Could you check a few things on this model? Use its own coordinates, in mm. Face numbers are marked on the shaded views. A direction names the side the tool comes from. Round coordinates to 2 decimals unless told otherwise and drop trailing zeros. Loops run counter-clockwise (first coordinate to the right, second up) from the corner with the lowest first, then second, coordinate; pieces in that order, holes last.
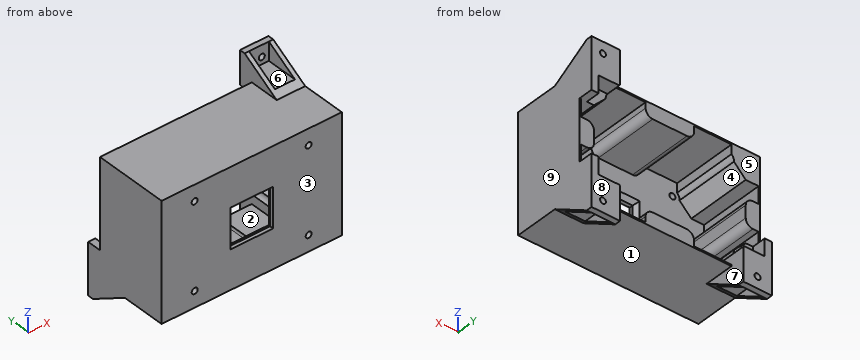
from build123d import *

# Parameters (mm, degrees)
SKETCH_1_W               = 126.5
SKETCH_1_H               = 82.5
SKETCH_1_R               = 2.1
SKETCH_1_W_2             = 30
SKETCH_1_H_2             = 28
EXTRUDE_2_DEPTH          = 6
CHAMFER_1_SIZE           = 2
CHAMFER_1_SIZE2          = 3.464101615
SKETCH_2_W               = 34
SKETCH_2_H               = 10
SKETCH_2_W_2             = 10
SKETCH_2_H_2             = 18.59934511
SKETCH_2_W_3             = 1
SKETCH_2_H_3             = 11.900654894
SKETCH_2_H_4             = 18.599345106
SKETCH_2_H_5             = 12
SKETCH_2_W_4             = 26.25
SKETCH_2_H_6             = 1
SKETCH_2_H_7             = 11.999999996
EXTRUDE_3_DEPTH          = 46
EXTRUDE_4_DEPTH          = 10
EXTRUDE_7_DEPTH          = 20
EXTRUDE_8_DEPTH          = 20
CUT_EXTRUDE_1_DEPTH      = 205.414906938
CUT_EXTRUDE_1_DEPTH_BACK = 205.414906938
SKETCH_6_R               = 2.1
SKETCH_7_W               = 14
SKETCH_7_H               = 13.763943164
SKETCH_7_H_2             = 13.67346934
SKETCH_7_H_3             = 14.015580363
SKETCH_7_H_4             = 13.891937121
CUT_EXTRUDE_2_DEPTH      = 58
FILLET_1_R               = 5
SKETCH_9_R               = 5
CUT_EXTRUDE_4_DEPTH      = 203.675736531


with BuildPart() as part:
    # Эскиз1 → Бобышка-Вытянуть2 (new body)
    with BuildSketch(Plane(origin=(0, 77.195974268, 0), x_dir=(1, 0, 0), z_dir=(0, 1, 0))):
        with Locations((64.808980694, -89.523129836)):
            Rectangle(SKETCH_1_W, SKETCH_1_H)
        with Locations(Location((24.808980694, -59.523129836, 0), (0, 0, 180))):
            Circle(SKETCH_1_R, mode=Mode.SUBTRACT)
        with Locations(Location((104.808980694, -59.523129836, 0), (0, 0, 180))):
            Circle(SKETCH_1_R, mode=Mode.SUBTRACT)
        with Locations(Location((104.808980694, -119.523129836, 0), (0, 0, 180))):
            Circle(SKETCH_1_R, mode=Mode.SUBTRACT)
        with Locations(Location((24.808980694, -119.523129836, 0), (0, 0, 180))):
            Circle(SKETCH_1_R, mode=Mode.SUBTRACT)
        with Locations((64.808980694, -89.523129836)):
            Rectangle(SKETCH_1_W_2, SKETCH_1_H_2, mode=Mode.SUBTRACT)
    extrude(amount=EXTRUDE_2_DEPTH)

    # Фаска1
    chamfer_1_edges = [part.edges().sort_by_distance(p)[0] for p in [
        (49.808980694, 83.195974268, 89.523129836),
        (64.808980694, 83.195974268, 103.523129836),
        (79.808980694, 83.195974268, 89.523129836),
        (64.808980694, 83.195974268, 75.523129836),
    ]]
    chamfer_1_side = [part.faces().sort_by_distance(p)[0] for p in [
        (64.808980694, 83.195974268, 49.78337816),
    ]]
    chamfer(chamfer_1_edges, length=CHAMFER_1_SIZE, length2=CHAMFER_1_SIZE2, reference=chamfer_1_side[0])

    # Эскиз2 → Бобышка-Вытянуть3 (add)
    with BuildSketch(Plane(origin=(0, 83.195974268, 0), x_dir=(1, 0, 0), z_dir=(0, 1, 0))):
        Polygon((1.558980694, -68.273129836), (11.558980694, -68.273129836), (21.558980694, -58.273129836), (21.558980694, -48.273129836), (1.558980694, -48.273129836), align=None)
        with Locations((64.808980694, -53.273129836)):
            Rectangle(SKETCH_2_W, SKETCH_2_H)
        Polygon((118.058980694, -68.273129836), (108.058980694, -58.273129836), (108.058980694, -48.273129836), (128.058980694, -48.273129836), (128.058980694, -68.273129836), align=None)
        with Locations((123.058980694, -89.473457285)):
            Rectangle(SKETCH_2_W_2, SKETCH_2_H_2)
        Polygon((108.058980694, -120.773129836), (118.058980694, -110.773129836), (128.058980694, -110.773129836), (128.058980694, -130.773129836), (108.058980694, -130.773129836), align=None)
        with Locations((64.808980694, -125.773129836)):
            Rectangle(SKETCH_2_W, SKETCH_2_H)
        Polygon((21.558980694, -130.773129836), (21.558980694, -120.773129836), (11.558980694, -110.773129836), (1.558980694, -110.773129836), (1.558980694, -130.773129836), align=None)
        with Locations((2.058980694, -74.223457283)):
            Rectangle(SKETCH_2_W_3, SKETCH_2_H_3)
        with Locations((6.558980694, -89.473457283)):
            Rectangle(SKETCH_2_W_2, SKETCH_2_H_4)
        with Locations((2.058980694, -104.773129836)):
            Rectangle(SKETCH_2_W_3, SKETCH_2_H_5)
        with Locations((34.683980694, -130.273129836)):
            Rectangle(SKETCH_2_W_4, SKETCH_2_H_6)
        with Locations((94.933980694, -130.273129836)):
            Rectangle(SKETCH_2_W_4, SKETCH_2_H_6)
        with Locations((127.558980694, -104.773129838)):
            Rectangle(SKETCH_2_W_3, SKETCH_2_H_7)
        with Locations((127.558980694, -74.223457283)):
            Rectangle(SKETCH_2_W_3, SKETCH_2_H_3)
        with Locations((94.933980694, -48.773129836)):
            Rectangle(SKETCH_2_W_4, SKETCH_2_H_6)
        with Locations((34.683980694, -48.773129836)):
            Rectangle(SKETCH_2_W_4, SKETCH_2_H_6)
    extrude(amount=EXTRUDE_3_DEPTH)

    # Эскиз3 → Бобышка-Вытянуть4 (add)
    with BuildSketch(Plane(origin=(0, 129.195974268, 0), x_dir=(1, 0, 0), z_dir=(0, 1, 0))):
        Polygon((6.558980694, -68.273129836), (6.558980694, -56.273129836), (21.558980694, -56.273129836), (21.558980694, -48.273129836), (1.558980694, -48.273129836), (1.558980694, -68.273129836), align=None)
        Polygon((123.058980694, -68.273129836), (123.058980694, -56.273129836), (108.058980694, -56.273129836), (108.058980694, -48.273129836), (128.058980694, -48.273129836), (128.058980694, -68.273129836), align=None)
        Polygon((123.058980694, -110.773129836), (123.058980694, -122.773129836), (108.058980694, -122.773129836), (108.058980694, -130.773129836), (128.058980694, -130.773129836), (128.058980694, -110.773129836), align=None)
    extrude(amount=EXTRUDE_4_DEPTH)

    # Эскиз4 → Бобышка-Вытянуть7 (add)
    with BuildSketch(Plane.ZY.offset(-1.558980694)):
        Polygon((48.273129836, 139.195974268), (48.273129836, 108.195974268), (32.273129836, 135.145974268), (32.273129836, 139.195974268), align=None)
    extrude(amount=-EXTRUDE_7_DEPTH)

    # Эскиз5 → Бобышка-Вытянуть8 (add)
    with BuildSketch(Plane(origin=(128.058980694, 0, 0), x_dir=(0, 0, -1), z_dir=(1, 0, 0))):
        Polygon((-130.773129836, 139.195974268), (-130.773129836, 108.145974268), (-146.773129836, 135.145974268), (-146.773129836, 139.195974268), align=None)
        Polygon((-48.273129836, 139.195974268), (-48.273129836, 108.195974268), (-32.273129836, 135.145974268), (-32.273129836, 139.195974268), align=None)
    extrude(amount=-EXTRUDE_8_DEPTH)

    # Эскиз6 → Вырез-Вытянуть1 (cut, two sides: drawn at the far end of the back side and taken through both)
    with BuildSketch(Plane(origin=(0, 139.195974268, 0), x_dir=(1, 0, 0), z_dir=(0, 1, 0)).offset(-CUT_EXTRUDE_1_DEPTH_BACK)):
        with Locations(Location((120.058980694, -40.273129836, 0), (0, 0, 90))):
            Circle(SKETCH_6_R)
        with Locations(Location((11.55898069, -40.273129836, 0), (0, 0, 180))):
            Circle(SKETCH_6_R)
        with Locations((11.55898069, -138.773129836)):
            Circle(SKETCH_6_R)
        with Locations(Location((120.058980694, -138.773129836, 0), (0, 0, 180))):
            Circle(SKETCH_6_R)
    extrude(amount=CUT_EXTRUDE_1_DEPTH + CUT_EXTRUDE_1_DEPTH_BACK, mode=Mode.SUBTRACT)

    # Эскиз7 → Вырез-Вытянуть2 (cut)
    with BuildSketch(Plane(origin=(0, 77.195974268, 0), x_dir=(-1, 0, 0), z_dir=(0, -1, 0))):
        with Locations((-11.558980694, -38.391158254)):
            Rectangle(SKETCH_7_W, SKETCH_7_H)
        with Locations((-118.058980694, -38.436395166)):
            Rectangle(SKETCH_7_W, SKETCH_7_H_2)
        with Locations((-118.058980694, -140.780920018)):
            Rectangle(SKETCH_7_W, SKETCH_7_H_3)
        with Locations((-11.558980694, -140.719098397)):
            Rectangle(SKETCH_7_W, SKETCH_7_H_4)
    extrude(amount=-CUT_EXTRUDE_2_DEPTH, mode=Mode.SUBTRACT)

    # Скругление1
    fillet_1_edges = [part.edges().sort_by_distance(p)[0] for p in [
        (81.808980694, 106.195974268, 120.773129836),
        (47.808980694, 106.195974268, 120.773129836),
        (11.558980694, 106.195974268, 98.773129836),
        (11.558980694, 106.195974268, 80.17378473),
        (47.808980694, 106.195974268, 58.273129836),
        (81.808980694, 106.195974268, 58.273129836),
        (118.058980694, 106.195974268, 80.17378473),
        (118.058980694, 106.195974268, 98.77312984),
    ]]
    fillet(fillet_1_edges, radius=FILLET_1_R)

    # Эскиз9 → Вырез-Вытянуть4 (cut, through all)
    with BuildSketch(Plane(origin=(0, 83.195974268, 0), x_dir=(1, 0, 0), z_dir=(0, 1, 0))):
        with Locations((24.808980694, -59.523129836)):
            Circle(SKETCH_9_R)
        with Locations((104.808980694, -59.523129836)):
            Circle(SKETCH_9_R)
        with Locations((104.808980694, -119.523129836)):
            Circle(SKETCH_9_R)
        with Locations((24.808980694, -119.523129836)):
            Circle(SKETCH_9_R)
    extrude(amount=CUT_EXTRUDE_4_DEPTH, mode=Mode.SUBTRACT)


solid = part.part
Item 1: If I drill on line 1 along X through (y, z) = (121, 73); line 2 along Z through (x, y) = (25.5, 109); line 3 along X through (y, z) = (126.5, 53), over which ranges is the centre line in solid material (lowest first)?
Results list:
line 1: x = 1.56 to 2.56, 127.06 to 128.06
line 2: z = 48.27 to 49.27, 129.77 to 130.77
line 3: x = 1.56 to 21.56, 47.81 to 81.81, 108.06 to 128.06
Item 2: For the marked faces 5, 6, 7, 8 and 9, which set-ups out of +Z, -Z, +X, -X, +Y, -Y let a thin tool reach every point of the face, with its end or its side?
Results list:
face 5: +Z, -X, +Y
face 6: +Z, -Y
face 7: +Y
face 8: +Z, -Z, +X, -X, +Y
face 9: +Z, -Z, +X, +Y, -Y
Item 3: If we section it at A-A, the plane z = 102: Please give me the cut outline in (x, y), then the cut area to 3 significant figures.
Results list:
outline: (1.56, 77.2) - (49.81, 77.2) - (49.81, 79.73) - (47.81, 83.2) - (2.56, 83.2) - (2.56, 129.2) - (1.56, 129.2) - close; (79.81, 77.2) - (128.06, 77.2) - (128.06, 129.2) - (127.06, 129.2) - (127.06, 83.2) - (81.81, 83.2) - (79.81, 79.73) - close
area: 664 mm2
Item 4: We'd pull the mould along Z, two halves only. Please class the marked faces 1, 2, 3 and 4: released by +Z, released by -Z, zero draft, split by the parting line, or undercut.
Results list:
face 1: released by -Z
face 2: undercut
face 3: zero draft
face 4: undercut
Item 5: If we section it at B-B, the plane x = 56.5: Please give me the cut outline in (y, z).
Results list:
outline: (77.2, 48.27) - (129.2, 48.27) - (129.2, 58.27) - (83.2, 58.27) - (83.2, 73.52) - (79.73, 75.52) - (77.2, 75.52) - close; (77.2, 103.52) - (79.73, 103.52) - (83.2, 105.52) - (83.2, 120.77) - (129.2, 120.77) - (129.2, 130.77) - (77.2, 130.77) - close
Item 6: Will these pins go through, and if not, where does the flat tip stop? pin 1 (6 mm diameter, centred on x = 96.5, y = 108, fed in from +Z); pin 2 (9.5 mm diameter, centred on x = 118.5, z = 114.5, fed in from +Y); pin 3 (11 mm diameter, centred on x = 125, y = 106, fed in from +Z); pin 4 (7 mm diameter, centred on x = 67, y = 115, fed in from -Z).
Results list:
pin 1: stops at z = 130.77
pin 2: stops at y = 139.2
pin 3: stops at z = 132.76
pin 4: stops at z = 48.27
Item 7: If we section it at C-C, the plane x = 29: Please give me the cut outline in (y, z).
Results list:
outline: (77.2, 48.27) - (129.2, 48.27) - (129.2, 49.27) - (83.2, 49.27) - (83.2, 129.77) - (129.2, 129.77) - (129.2, 130.77) - (77.2, 130.77) - close
Item 8: If we section it at D-D, the plane y = 132.5: Count the separate pieces of the cut face and the enclosed holes in it, then the cut area to 3 significant figures.
Results list:
separate pieces: 3
enclosed holes: 0
area: 1,050 mm2
